Design review of the part built by this model. Coordinates are the model's own, in mm. A direction names the side the tool comes from. Coordinates: 2 decimals unless noted, no trailing zeros. Write each loop counter-clockwise with the first axis right and the second up, starting at its lowest first coordinate (ties: lowest second). Pieces come first, ordered by that corner, then holes. Notation, with made-up numbers: (-9, -24.75) - (43, -24.75) arc R25 ccw to (43, 1.25) - close; hole circle Ø5 at (72, 10). An arc over 180 degrees is marked (long way). Answer as CSV lines item,"result". Start each with the question number.
Q1. Machinability: for faces 4 (the face through (-2, 41, 0)), 5 (the face through (1.6, 42, 53)), which of the approach directions +Z, -Z, +X, -X, +Y, -Y give a long, thin tool a straight path to every point of the face, cutting with its end or side? Answer none if there is none.
Q2. Clearance check with a flat-ended pin moving along its axis: pin 1 (1 mm diameter, centred on x = -2, z = 29, fed in from +Y). State where the tip first meets the part, or that it passes through.
Q3. We need section A-A (y = 62.5). Write out the cut boundary in (x, z), plus the area to 3 significant figures.
Q4. For line 1 along Z through (x, y) = (-1.75, 56); line 2 along X through (y, z) = (22, 52.5); line 3 along Y through (x, z) = (0.25, 29.5), list the stretches that pass through material, from the lowest coordinate up. Write a range as [from, to].
Q5. Mouldability with a two-part tool opening along Z and no side actions: class faces 1 (the face through (0, 80, 2)), 2 (the face through (2, 43, 4)), 3 (the face through (-2, 41, 55)) as pulls with the +Z half, pulls with the -Z half, needs draft (parallel to the pull), parting line crosses it, or undercut.
Autodesk Inventor part; units mm, degrees
ref_plane "YZ Plane" through (0, 0, 0) normal (1, 0, 0) x (0, 1, 0)
ref_plane "XZ Plane" through (0, 0, 0) normal (0, 1, 0) x (-1, 0, 0)
ref_plane "XY Plane" through (0, 0, 0) normal (0, 0, 1) x (1, 0, 0)
sketch "Эскиз1" plane through (0, 0, 0) normal (0, 0, 1) x (1, 0, 0)
  line L0 (0, 0) -> (0, 80)
  line L1 (0, 0) -> (0, 5)
  line L2 (0, 80) -> (0, 75)
  circle A0 centre (0, 75) radius 5
  circle A1 centre (0, 5) radius 5
  circle A2 centre (0, 5) radius 1.6
  circle A3 centre (0, 75) radius 1.6
  line L3 (-1.6, 75) -> (-1.6, 5)
  line L4 (1.6, 5) -> (1.6, 75)
  line L5 (-5, 75) -> (-5, 5)
  line L6 (5, 5) -> (5, 75)
  line L7 (-1.6, 9.7371) -> (1.6, 9.7371)
  circle A4 centre (0, 9.7371) radius 1.6
  point P0 (-1.6, 9.7371)
  dimension "d0" = 80
  dimension "d1" = 5
  dimension "d2" = 5
  dimension "d3" = 3.2
  dimension "d4" = 3.2
extrude "Выдавливание1" add sketch "Эскиз1" along normal blind 55 contours A1 L3 A2 L0 | L0 A2 L4 A1 | L5 A0 L3 A1 | A1 L4 A0 L6 | L3 A4 L0 A2 | A2 L0 A4 L4 | A0 L0 A3 L3 | A0 L4 A3 L0 picked at (-1.9727, 72.0221) picked at (1.9727, 72.0221)
ref_plane "РабПлоскость1" through (0, 0, 27.5) normal (0, 0, -1) x (-1, 0, 0)
sketch "Эскиз2" plane through (0, 0, 27.5) normal (0, 0, -1) x (-1, 0, 0)
  circle A0 centre (0, 5) radius 1.6
  circle A1 centre (0, 5) radius 5
  line L0 (-5, 5) -> (-5, 75)
  ellipse E0 centre (0, 5) end of major axis (-5, 5) minor radius 3.1371
  line L1 (5, 75) -> (5, 5)
  line L2 (5, 5) -> (-5, 5)
  line L3 (-5, 5) -> (-5, 83.8736)
  line L4 (-5, 83.8736) -> (5, 83.8736)
  line L5 (5, 83.8736) -> (5, 5)
  point P0 (0, 0)
extrude "Выдавливание2" cut sketch "Эскиз2" against normal mid plane 47 contours E0 A1 | A1 L0 L3 L4 L5 L1 picked at (-0.9942, 8.9185)
properties part number "arrow"
Results list:
1,face 4,"-Z, +X, -X, +Y, -Y"
1,face 5,"+Z, -Z"
2,pin 1,"stops at y = 7.99"
3,outline,"(-5, 0) - (-1.6, 0) - (-1.6, 4) - (-5, 4) - close; (-5, 51) - (-1.6, 51) - (-1.6, 55) - (-5, 55) - close; (1.6, 0) - (5, 0) - (5, 4) - (1.6, 4) - close; (1.6, 51) - (5, 51) - (5, 55) - (1.6, 55) - close"
3,area,"54.4 mm2"
4,line 1,"z = [0, 4], [51, 55]"
4,line 2,"x = [-5, -1.6], [1.6, 5]"
4,line 3,"y = [0.01, 3.42], [6.58, 8.13]"
5,face 1,"needs draft"
5,face 2,"undercut"
5,face 3,"pulls with the +Z half"
